```python
from build123d import *

# Parameters (mm, degrees)
SKETCH1_W           = 200
SKETCH1_H           = 200
BOSS_EXTRUDE1_DEPTH = 5
SKETCH2_R           = 2.5
CUT_EXTRUDE1_DEPTH  = 5
SKETCH3_R           = 1.5
CUT_EXTRUDE2_DEPTH  = 5
SKETCH4_R           = 21
CUT_EXTRUDE3_DEPTH  = 7


with BuildPart() as part:
    # Sketch1 → Boss-Extrude1 (new body)
    with BuildSketch(Plane(origin=(0, 0, 0), x_dir=(1, 0, 0), z_dir=(0, 1, 0))):
        Rectangle(SKETCH1_W, SKETCH1_H)
    extrude(amount=BOSS_EXTRUDE1_DEPTH)

    # Sketch2 → Cut-Extrude1 (cut)
    with BuildSketch(Plane(origin=(0, 5, 0), x_dir=(1, 0, 0), z_dir=(0, 1, 0))):
        with Locations(Location((77.781745931, 77.781745931, 0), (0, 0, 270))):
            Circle(SKETCH2_R)
        with Locations(Location((77.781745931, -77.781745931, 0), (0, 0, 270))):
            Circle(SKETCH2_R)
        with Locations(Location((-77.781745931, -77.781745931, 0), (0, 0, 270))):
            Circle(SKETCH2_R)
        with Locations(Location((-77.781745931, 77.781745931, 0), (0, 0, 270))):
            Circle(SKETCH2_R)
    extrude(amount=-CUT_EXTRUDE1_DEPTH, mode=Mode.SUBTRACT)

    # Sketch3 → Cut-Extrude2 (cut)
    with BuildSketch(Plane(origin=(0, 5, 0), x_dir=(1, 0, 0), z_dir=(0, 1, 0))):
        with Locations(Location((0, -45, 0), (0, 0, 270))):
            Circle(SKETCH3_R)
        with Locations(Location((-45, 0, 0), (0, 0, 270))):
            Circle(SKETCH3_R)
        with Locations(Location((0, 45, 0), (0, 0, 270))):
            Circle(SKETCH3_R)
        with Locations(Location((45, 0, 0), (0, 0, 270))):
            Circle(SKETCH3_R)
    extrude(amount=-CUT_EXTRUDE2_DEPTH, mode=Mode.SUBTRACT)

    # Sketch4 → Cut-Extrude3 (cut)
    with BuildSketch(Plane(origin=(0, 5, 0), x_dir=(1, 0, 0), z_dir=(0, 1, 0))):
        with Locations(Location((0, 0, 0), (0, 0, 270))):
            Circle(SKETCH4_R)
    extrude(amount=-CUT_EXTRUDE3_DEPTH, mode=Mode.SUBTRACT)


solid = part.part
```
For this review, take the finished solid that the model builds, in its own axes (mm). Coordinates: 2 decimals unless noted, no trailing zeros. Loops run counter-clockwise (first coordinate to the right, second up) from the corner with the lowest first, then second, coordinate; pieces in that order, holes last. Notation, with made-up numbers: (29, 79) - (85, 79) arc R9 ccw to (85, 89) - close; hole circle Ø6 at (10.25, 80). An arc over 180 degrees is marked (long way). Use one line per item in the form item = value. Start each with the question number.
1) Take a section at A-A (x = -10). State the section outline as (y, z) points, plus the area to 3 significant figures.
2) For pin 1 (4.5 mm diameter, centred on x = -77.78, z = -77.78, fed in from +Y), flat-tipped, find the tip position at first contact; note if it passes through.
3) Draft analysis for pull direction Z (two halves, no side actions). For faces 1 (the face through (-1, 2, -100)), 2 (the face through (-1, 5, -24)), 3 (the face through (6.31, 2.54, 20.03)), state which applies: released by +Z, released by -Z, zero draft, split by the parting line, or undercut.
4) To check wall thickness, follow probe 1 along X at (y, z) = (4.4, -77.5); probe 2 along X at (y, z) = (1, 45); probe 3 along X at (y, z) = (3.55, 0). State the ranges of each line that lie inside material, in increasing order. Write a range as from..to.
5) Take a section at B-B (y = 1.7). State how many separate pieces and enclosed holes the cut face has, plus the area to 3 significant figures.
From the geometry:
q1.outline = (0, -100) - (5, -100) - (5, -18.47) - (0, -18.47) - close; (0, 18.47) - (5, 18.47) - (5, 100) - (0, 100) - close
q1.area = 815 mm2
q2.pin_1 = through
q3.face_1 = released by -Z
q3.face_2 = zero draft
q3.face_3 = undercut
q4.probe_1 = -100..-80.27, -75.3..75.3, 80.27..100
q4.probe_2 = -100..-1.5, 1.5..100
q4.probe_3 = -100..-46.5, -43.5..-21, 21..43.5, 46.5..100
q5.separate_pieces = 1
q5.enclosed_holes = 9
q5.area = 38,500 mm2
